Autodesk Fusion 360 part; units mm, degrees
sketch "Sketch1" plane through (0, 0, 0) normal (0, 0, 1) x (1, 0, 0)
  line L0 (0, 0) -> (44, 0)
  line L1 (44, 0) -> (44, -8)
  line L2 (44, -8) -> (0, -8)
  line L3 (0, -8) -> (0, 0)
  line L4 (44, -8) -> (34, -8)
  line L5 (34, -8) -> (34, -28)
  line L6 (34, -28) -> (44, -28)
  line L7 (44, -28) -> (44, -8)
  circle A0 centre (2.5, -2.5) radius 1.5
  line L8 (2.5, -2.5) -> (2.5, 0) construction
  line L9 (2.5, -2.5) -> (0, -2.5) construction
  line L10 (13.5, -8) -> (17.5, -8)
  line L11 (17.5, -8) -> (17.5, -6)
  line L12 (17.5, -6) -> (13.5, -6)
  line L13 (13.5, -6) -> (13.5, -8)
  point P0 (15.5, -6)
  dimension "d1" = 3
  dimension "d2" = 2.5
  dimension "d3" = 8
  dimension "d4" = 13
  dimension "d5" = 2
  dimension "d6" = 4
  dimension "d7" = 44
  dimension "d9" = 20
  dimension "d23" = 34
extrude "Extrude1" add sketch "Sketch1" along normal blind 2 contours L0 L1 L2 L3 L4 L11 L12 L13 | L2 L4 L5 L6 L7
extrude "Extrude2" add sketch "Sketch1" along normal blind 10 contours L2 L4 L5 L6 L7
fillet "Fillet1" radius 2.5 3 edges at (0, 0, 1) (0, -8, 1) (44, 0, 1)
sketch "Sketch2" plane through (0, -28, 0) normal (0, -1, 0) x (1, 0, 0)
  line L0 (34, 0) -> (44, 0)
  line L1 (44, 0) -> (44, 10)
  line L2 (44, 10) -> (34, 10)
  line L3 (34, 10) -> (34, 0)
  line L4 (34, 10) -> (44, 0) construction
  line L5 (36, 3.5) -> (42, 6.5) construction
  line L6 (36, 3.5) -> (42, 3.5)
  line L7 (42, 3.5) -> (42, 6.5)
  line L8 (42, 6.5) -> (36, 6.5)
  line L9 (36, 6.5) -> (36, 3.5)
  dimension "d17" = 6
  dimension "d18" = 3
extrude "Extrude3" cut sketch "Sketch2" against normal through all contours L6 L7 L8 L9
sketch "Sketch3" plane through (0, 0, 10) normal (0, 0, 1) x (-1, 0, 0)
  line L0 (-44, 28) -> (-44, 8)
  line L1 (-44, 8) -> (-34, 8)
  line L2 (-34, 8) -> (-34, 28)
  line L3 (-34, 28) -> (-44, 28)
  line L4 (-34, 8) -> (-44, 28) construction
  circle A0 centre (-39, 18) radius 1.75
  dimension "d20" = 3.5
extrude "Extrude4" cut sketch "Sketch3" against normal up to surface (6.5 mm away) contours A0
Verification items for the finished model (mm, model axes). A direction names the side the tool comes from. Round coordinates to 2 decimals unless told otherwise and drop trailing zeros. Write each loop counter-clockwise with the first axis right and the second up, starting at its lowest first coordinate (ties: lowest second). Pieces come first, ordered by that corner, then holes.
(1) Mould release check, pull along X, two halves, no side actions. Record for faces 1 (the flat face through (44, -18, 5)), 2 (the cylindrical face through (2.175, -1.036, 0.986)), 3 (the flat face through (41, -18, 10)): pulls with the +X half, pulls with the -X half, needs draft (parallel to the pull), parting line crosses it, or undercut.
Returned:
face 1: pulls with the +X half
face 2: undercut
face 3: needs draft
(2) Depth check by flat-ended pin: pin 1 Ø4 at (x, y) = (2.5, -2.5) entering from +Z; pin 2 Ø1 at (x, z) = (27, 0.5) entering from -Y; pin 3 Ø5 at (y, z) = (-21, 6.5) entering from -X. Enter the tip coordinate at first touch or a pass-through.
Returned:
pin 1: stops at z = 2
pin 2: stops at y = -8
pin 3: stops at x = 34
(3) Access from +Z, -Z, +X, -X, +Y, -Y to the whole of each face (thin tool, end or side, straight path). Record for faces 4 (the flat face through (39, -8, 7)), 5 (the flat face through (41, -18, 6.5)), 6 (the cylindrical face through (43.287, -0.752, 1.014)), 7 (the flat face through (8, -8, 1)), 8 (the flat face through (17.5, -7, 1)).
Returned:
face 4: +Z, +X, -X, +Y
face 5: +Y, -Y
face 6: +Z, -Z, +X, +Y
face 7: +Z, -Z, -X, -Y
face 8: +Z, -Z, -Y
(4) Section check D-D (z = 5). Enter the section's corners in (x, y), plus the area to 3 significant figures.
Returned:
outline: (34, -28) - (36, -28) - (36, -8) - (34, -8) - close; (42, -28) - (44, -28) - (44, -8) - (42, -8) - close
area: 80.0 mm2
(5) Section check B-B (x = 39). Enter the section's corners in (y, z).
Returned:
outline: (-28, 0) - (0, 0) - (0, 2) - (-8, 2) - (-8, 3.5) - (-28, 3.5) - close; (-28, 6.5) - (-19.75, 6.5) - (-19.75, 10) - (-28, 10) - close; (-16.25, 6.5) - (-8, 6.5) - (-8, 10) - (-16.25, 10) - close
(6) Section check C-C (y = -8.5). Enter the section's corners in (x, z).
Returned:
outline: (34, 0) - (44, 0) - (44, 10) - (34, 10) - close; hole (36, 3.5) - (42, 3.5) - (42, 6.5) - (36, 6.5) - close
(7) Section check A-A (z = 1). Enter the section's corners in (x, y), plus the area to 3 significant figures.
Returned:
outline: (0, -5.5) arc R2.5 ccw to (2.5, -8) - (13.5, -8) - (13.5, -6) - (17.5, -6) - (17.5, -8) - (34, -8) - (34, -28) - (44, -28) - (44, -2.5) arc R2.5 ccw to (41.5, 0) - (2.5, 0) arc R2.5 ccw to (0, -2.5) - close; hole circle Ø3 at (2.5, -2.5)
area: 533 mm2
(8) Material ranges on line 1 (X direction, y = -11.25, z = 4.75); line 2 (Y direction, x = 39, z = 7.45); line 3 (X direction, y = -18, z = 7.35), recorded low to high.
Returned:
line 1: x = 34 to 36, 42 to 44
line 2: y = -28 to -19.75, -16.25 to -8
line 3: x = 34 to 37.25, 40.75 to 44
